For this review, take the finished solid that the model builds, in its own axes (mm). Face numbers are marked on the shaded views. Coordinates: 2 decimals unless noted, no trailing zeros. Loops run counter-clockwise (first coordinate to the right, second up) from the corner with the lowest first, then second, coordinate; pieces in that order, holes last. Notation, with made-up numbers: (40, 58) -> (71, 58) arc R20 cw to (71, 81) -> close; hole circle Ø3 at (-37.75, 54.5). An arc over 180 degrees is marked (long way). Use a Markdown table: item, result.
from build123d import *

# Parameters (mm, degrees)
SKETCH1_R           = 61
SKETCH1_R_2         = 56
BOSS_EXTRUDE1_DEPTH = 300
SKETCH3_R           = 56
BOSS_EXTRUDE2_DEPTH = 5
CUT_EXTRUDE1_REACH  = 294.988
SKETCH4_R           = 1.5
SKETCH5_R           = 56
BOSS_EXTRUDE3_DEPTH = 5
CUT_EXTRUDE2_REACH  = 309.355
SKETCH6_W           = 12.82
SKETCH6_H           = 30.34


with BuildPart() as part:
    # Sketch1 → Boss-Extrude1 (new body)
    with BuildSketch(Plane(origin=(0, 0, 0), x_dir=(1, 0, 0), z_dir=(0, 1, 0))):
        with Locations(Location((0, 0, 0), (0, 0, 270))):
            Circle(SKETCH1_R)
        with Locations(Location((0, 0, 0), (0, 0, 270))):
            Circle(SKETCH1_R_2, mode=Mode.SUBTRACT)
    extrude(amount=BOSS_EXTRUDE1_DEPTH)

    # Sketch3 → Boss-Extrude2 (add)
    with BuildSketch(Plane(origin=(0, 20, 0), x_dir=(1, 0, 0), z_dir=(0, 1, 0))):
        with Locations(Location((0, 0, 0), (0, 0, 270))):
            Circle(SKETCH3_R)
    extrude(amount=BOSS_EXTRUDE2_DEPTH)

    # Sketch4 → Cut-Extrude1 (cut, up to next)
    with BuildSketch(Plane.XZ.offset(-20), mode=Mode.PRIVATE) as cut_extrude1_sk1:
        with Locations(Location((10, 0, 0), (0, 0, 270))):
            Circle(SKETCH4_R)
    cut_extrude1_tool1 = extrude(cut_extrude1_sk1.sketch, amount=-CUT_EXTRUDE1_REACH, mode=Mode.PRIVATE) & part.part
    # Sketch4 → Cut-Extrude1 (cut, up to next)
    with BuildSketch(Plane.XZ.offset(-20), mode=Mode.PRIVATE) as cut_extrude1_sk2:
        with Locations(Location((0, 10, 0), (0, 0, 270))):
            Circle(SKETCH4_R)
    cut_extrude1_tool2 = extrude(cut_extrude1_sk2.sketch, amount=-CUT_EXTRUDE1_REACH, mode=Mode.PRIVATE) & part.part
    # Sketch4 → Cut-Extrude1 (cut, up to next)
    with BuildSketch(Plane.XZ.offset(-20), mode=Mode.PRIVATE) as cut_extrude1_sk3:
        with Locations(Location((-10, 0, 0), (0, 0, 270))):
            Circle(SKETCH4_R)
    cut_extrude1_tool3 = extrude(cut_extrude1_sk3.sketch, amount=-CUT_EXTRUDE1_REACH, mode=Mode.PRIVATE) & part.part
    # Sketch4 → Cut-Extrude1 (cut, up to next)
    with BuildSketch(Plane.XZ.offset(-20), mode=Mode.PRIVATE) as cut_extrude1_sk4:
        with Locations(Location((0, -10, 0), (0, 0, 270))):
            Circle(SKETCH4_R)
    cut_extrude1_tool4 = extrude(cut_extrude1_sk4.sketch, amount=-CUT_EXTRUDE1_REACH, mode=Mode.PRIVATE) & part.part
    add(cut_extrude1_tool1.solids().sort_by_distance((10, 20, 0))[0], mode=Mode.SUBTRACT)
    add(cut_extrude1_tool2.solids().sort_by_distance((0, 20, 10))[0], mode=Mode.SUBTRACT)
    add(cut_extrude1_tool3.solids().sort_by_distance((-10, 20, 0))[0], mode=Mode.SUBTRACT)
    add(cut_extrude1_tool4.solids().sort_by_distance((0, 20, -10))[0], mode=Mode.SUBTRACT)

    # Sketch5 → Boss-Extrude3 (add)
    with BuildSketch(Plane(origin=(0, 290, 0), x_dir=(1, 0, 0), z_dir=(0, 1, 0))):
        with Locations(Location((0, 0, 0), (0, 0, 270))):
            Circle(SKETCH5_R)
    extrude(amount=BOSS_EXTRUDE3_DEPTH)

    # Sketch6 → Cut-Extrude2 (cut, up to next)
    with BuildSketch(Plane(origin=(0, 295, 0), x_dir=(1, 0, 0), z_dir=(0, 1, 0)), mode=Mode.PRIVATE) as cut_extrude2_sk1:
        Rectangle(SKETCH6_W, SKETCH6_H)
    cut_extrude2_tool1 = extrude(cut_extrude2_sk1.sketch, amount=-CUT_EXTRUDE2_REACH, mode=Mode.PRIVATE) & part.part
    add(cut_extrude2_tool1.solids().sort_by_distance((0, 295, 0))[0], mode=Mode.SUBTRACT)


solid = part.part
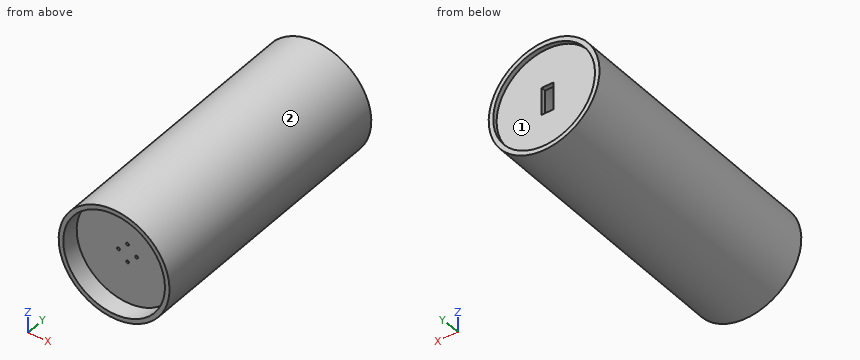
(1) For pin 1 Ø2 at (x, z) = (-38.5, 19) entering from +Y; pin 2 Ø4 at (x, z) = (0, -10) entering from -Y; pin 3 Ø4 at (x, y) = (2.5, 291.5) entering from +Z, all flat-tipped, find the tip position at first contact; note any pin that passes through.
Found:
| item | result |
|---|---|
| pin 1 | stops at y = 295 |
| pin 2 | stops at y = 20 |
| pin 3 | stops at z = 61 |
(2) For line 1 along X through (y, z) = (23, 0); line 2 along X through (y, z) = (7.25, 0); line 3 along Y through (x, z) = (10, -12), list the stretches that pass through material, from the lowest coordinate up.
Found:
| item | result |
|---|---|
| line 1 | x = -61 to -11.5, -8.5 to 8.5, 11.5 to 61 |
| line 2 | x = -61 to -56, 56 to 61 |
| line 3 | y = 20 to 25, 290 to 295 |
(3) Mouldability with a two-part tool opening along X and no side actions: class the marked faces 1 and 2 as pulls with the +X half, pulls with the -X half, needs draft (parallel to the pull), parting line crosses it, or undercut.
Found:
| item | result |
|---|---|
| face 1 | undercut |
| face 2 | parting line crosses it |
(4) Take a section at C-C on y = 74. Write out the cut boundary in (x, z).
Found:
| item | result |
|---|---|
| outline | circle Ø122 at (0, 0); hole circle Ø112 at (0, 0) |
(5) Take a section at B-B on x = 20. Write out the cut boundary in (y, z), plus the area to 3 significant figures.
Found:
| item | result |
|---|---|
| outline | (0, -57.63) -> (300, -57.63) -> (300, -52.31) -> (295, -52.31) -> (295, 52.31) -> (300, 52.31) -> (300, 57.63) -> (0, 57.63) -> (0, 52.31) -> (20, 52.31) -> (20, -52.31) -> (0, -52.31) -> close; hole (25, -52.31) -> (290, -52.31) -> (290, 52.31) -> (25, 52.31) -> close |
| area | 4,240 mm^2 |
(6) Take a section at A-A on z = -28. Write out the cut boundary in (x, y).
Found:
| item | result |
|---|---|
| outline | (-54.19, 0) -> (-48.5, 0) -> (-48.5, 20) -> (48.5, 20) -> (48.5, 0) -> (54.19, 0) -> (54.19, 300) -> (48.5, 300) -> (48.5, 295) -> (-48.5, 295) -> (-48.5, 300) -> (-54.19, 300) -> close; hole (-48.5, 25) -> (48.5, 25) -> (48.5, 290) -> (-48.5, 290) -> close |
